CAD build for the part. Positions are in the model's coordinates, mm. Give positions to 0.01 mm unless a question says otherwise; leave off trailing zeros. Loops run counter-clockwise (first coordinate to the right, second up) from the corner with the lowest first, then second, coordinate; pieces in that order, holes last. Notation, with made-up numbers: (87, 50.25) - (129, 50.25) arc R9 cw to (129, 63.25) - close; hole circle Ø9 at (-15.75, -1.5). An arc over 180 degrees is marked (long way). Return JSON: item names as keys, results as strings.
from build123d import *

# Parameters (mm, degrees)
EXTRUDE_1_DEPTH     = 6.28
SKETCH_2_OUTSIDE_W  = 22.412
SKETCH_2_OUTSIDE_H  = 20.482
SKETCH_2_OUTSIDE_R  = 6.235382907
CUT_EXTRUDE_2_DEPTH = 1
CUT_EXTRUDE_2_DRAFT = -45
SKETCH_3_OUTSIDE_W  = 22.412
SKETCH_3_OUTSIDE_H  = 20.482
SKETCH_3_OUTSIDE_R  = 6.235382907
CUT_EXTRUDE_3_DEPTH = 1
CUT_EXTRUDE_3_DRAFT = -45
SKETCH_4_R          = 3.4
CUT_EXTRUDE_4_DEPTH = 7.28
FILLET_1_R          = 1
FILLET_2_R          = 1


with BuildPart() as part:
    # Эскиз1 → Бобышка-Вытянуть1 (new body)
    with BuildSketch(Plane(origin=(0, 0, 0), x_dir=(1, 0, 0), z_dir=(0, 1, 0))):
        Polygon((7.2, 0), (3.6, 6.235382907), (-3.6, 6.235382907), (-7.2, 0), (-3.6, -6.235382907), (3.6, -6.235382907), align=None)
    extrude(amount=EXTRUDE_1_DEPTH)


with BuildPart() as cut_extrude_2_tool:
    # Эскиз2 outside → Вырез-Вытянуть2 (with draft: the straight prism first)
    with BuildSketch(Plane(origin=(0, 6.28, 0), x_dir=(1, 0, 0), z_dir=(0, 1, 0))):
        Rectangle(SKETCH_2_OUTSIDE_W, SKETCH_2_OUTSIDE_H)
        Circle(SKETCH_2_OUTSIDE_R, mode=Mode.SUBTRACT)
    extrude(amount=-CUT_EXTRUDE_2_DEPTH)
    # Вырез-Вытянуть2: the draft: its side faces are tilted about the plane it starts from
    cut_extrude_2_sides = [cut_extrude_2_tool.faces().sort_by_distance(p)[0] for p in [
        (0, 5.78, 10.241),
        (11.206, 5.78, 0),
        (0, 5.78, -10.241),
        (-11.206, 5.78, 0),
        (-6.235382907, 5.78, 0),
    ]]
    draft(cut_extrude_2_sides, Plane(origin=(0, 6.28, 0), x_dir=(1, 0, 0), z_dir=(0, 1, 0)), CUT_EXTRUDE_2_DRAFT)


with BuildPart() as part_1:
    add(part.part)

    # Вырез-Вытянуть2: cut by cut_extrude_2_tool
    add(cut_extrude_2_tool.part, mode=Mode.SUBTRACT)


with BuildPart() as cut_extrude_3_tool:
    # Эскиз3 outside → Вырез-Вытянуть3 (with draft: the straight prism first)
    with BuildSketch(Plane.XZ):
        Rectangle(SKETCH_3_OUTSIDE_W, SKETCH_3_OUTSIDE_H)
        Circle(SKETCH_3_OUTSIDE_R, mode=Mode.SUBTRACT)
    extrude(amount=-CUT_EXTRUDE_3_DEPTH)
    # Вырез-Вытянуть3: the draft: its side faces are tilted about the plane it starts from
    cut_extrude_3_sides = [cut_extrude_3_tool.faces().sort_by_distance(p)[0] for p in [
        (0, 0.5, -10.241),
        (11.206, 0.5, 0),
        (0, 0.5, 10.241),
        (-11.206, 0.5, 0),
        (-6.235382907, 0.5, 0),
    ]]
    draft(cut_extrude_3_sides, Plane.XZ, CUT_EXTRUDE_3_DRAFT)


with BuildPart() as part_2:
    add(part_1.part)

    # Вырез-Вытянуть3: cut by cut_extrude_3_tool
    add(cut_extrude_3_tool.part, mode=Mode.SUBTRACT)

    # Эскиз4 → Вырез-Вытянуть4 (cut, through all)
    with BuildSketch(Plane(origin=(0, 6.28, 0), x_dir=(1, 0, 0), z_dir=(0, 1, 0))):
        with Locations(Location((0, 0, 0), (0, 0, 270))):  # turned: the seam where the file's is
            Circle(SKETCH_4_R)
    extrude(amount=-CUT_EXTRUDE_4_DEPTH, mode=Mode.SUBTRACT)

    # Скругление1
    fillet_1_edges = [part_2.edges().sort_by_distance(p)[0] for p in [
        (0, 6.28, -3.4),
    ]]
    fillet(fillet_1_edges, radius=FILLET_1_R)

    # Скругление2
    fillet_2_edges = [part_2.edges().sort_by_distance(p)[0] for p in [
        (0, 0, -3.4),
    ]]
    fillet(fillet_2_edges, radius=FILLET_2_R)


solid = part_2.part
1. Pull direction Z, two halves, no side cores. Call faces 1 (the face through (6.465, 0.23, -0.016)), 2 (the face through (-3.32, 3.17, -0.74)), 3 (the face through (3, 0, 4)): +Z half, -Z half, draft (parallel to the pull), parting line (faces both ways), or undercut.
Values follow:
{"face 1": "parting line", "face 2": "undercut", "face 3": "draft"}
2. Drop a flat-ended pin along its axis: P1, Ø3, axis at y = 3.5, z = -2.5, coming from the +X side. Give the stop position or say it passes through.
Values follow:
{"P1": "stops at x = 6.62"}
3. Cut at A-A, the plane y = 4.75. Write the cut outline in (x, z), plus the area to 3 significant figures.
Values follow:
{"outline": "(-7.2, 0) - (-3.6, -6.24) - (3.6, -6.24) - (7.2, 0) - (3.6, 6.24) - (-3.6, 6.24) - close; hole circle Ø6.8 at (0, 0)", "area": "98.4 mm²"}
4. Drill centre lines: probe 1 along Z at (x, y) = (-2, 5.25); probe 2 along X at (y, z) = (6, 0.25); probe 3 along Z at (x, y) = (3, 0.5). Where is each one in solid material? Low to high.
Values follow:
{"probe 1": "z = -6.24 to -2.75, 2.75 to 6.24", "probe 2": "x = -6.51 to -3.7, 3.7 to 6.51", "probe 3": "z = -6.03 to -1.87, 1.87 to 6.03"}
